Input: part model. Units: mm. Frame: model coordinates. A direction names the side the tool comes from. Give positions to 0.01 mm unless a question says otherwise; leave off trailing zeros. One line per item, written item: value.
Autodesk Fusion 360 part; units mm, degrees
sketch "Sketch1" plane through (0, 0, 0) normal (0, 1, 0) x (1, 0, 0)
  circle A0 centre (0, 0) radius 13
  circle A1 centre (0, 0) radius 3
  line L0 (0, 0) -> (0, 10)
  line L1 (0, 10) -> (3, 10)
  line L2 (3, 10) -> (3, 12)
  line L3 (3, 12) -> (-3, 12)
  line L4 (-3, 12) -> (-3, 10)
  line L5 (-3, 10) -> (3, 10)
  line L6 (-3, 10) -> (3, 10)
  line L7 (3, 10) -> (3, 6)
  line L8 (3, 6) -> (-3, 6)
  line L9 (-3, 6) -> (-3, 10)
  dimension "d1" = 26
  dimension "d2" = 6
extrude "Extrude1" add sketch "Sketch1" along normal blind 1 contours L0 L5 L6 L8 L9 | L0 L1 L5 L6 L7 L8
extrude "Extrude2" add sketch "Sketch1" along normal blind 6 contours L1 L2 L3 L4 L5 L6
extrude "Extrude3" add 1 faces at (-1, 6, -11.3333) along direction (0, 1, 0) blind 1
sketch "Sketch2" plane through (0, 0, -10) normal (0, 0, 1) x (1, 0, 0)
  line L0 (-3, 1) -> (3, 1)
  line L1 (3, 1) -> (3, 7)
  line L2 (3, 7) -> (-3, 7)
  line L3 (-3, 7) -> (-3, 1)
  line L4 (0, 7) -> (0, 5)
  circle A0 centre (0, 5) radius 0.5
  circle A1 centre (0, 5) radius 3
  circle A2 centre (0, 5) radius 1.5
  dimension "d9" = 2
  dimension "d10" = 1
  dimension "d23" = 3
extrude "Extrude4" cut sketch "Sketch2" against normal blind 5.8 contours A0
extrude "Extrude5" add 1 faces at (1, 1, -7.3333) along direction (0, 1, 0) blind 1
extrude "Extrude6" cut 1 faces at (1, 2, -7.3333) along direction (0, -1, 0) blind 0.5
extrude "Extrude7" cut sketch "Sketch2" against normal blind 1 contours A2 | L2 A1 picked at (-0.9591, 6.7853)
fillet "Fillet1" radius 2.3 1 edges at (0, 1.5, -10)
extrude "Extrude8" add 1 faces at (-0.0125, 6.4995, -11) along direction (0, 0, 1) blind 1
extrude "Extrude9" add 1 faces at (-1, 7, -10.6667) along direction (0, 1, 0) blind 1
extrude "Extrude10" cut sketch "Sketch2" against normal blind 1 contours A2
fillet "Fillet2" radius 3 2 edges at (-3, 8, -11) (3, 8, -11)
Item 1: Pin query (flat end, axial travel): P1, Ø1, axis at x = 0, z = -8.5, coming from the +Y side; P2, Ø1.8, axis at x = 0, y = 5, coming from the +Z side; P3, Ø3.5, axis at x = 0.5, y = 5.5, coming from the +Z side. Return the tip coordinate at first contact, or that it passes through.
Verdict:
P1: stops at y = 1.54
P2: stops at z = -11
P3: stops at z = -10
Item 2: Access query for faces 4 (the face through (0, 0, -9)), 5 (the face through (0, 1.5, -7)), 6 (the face through (-1.5, 5.07, -10.49)). Directions: +Z, -Z, +X, -X, +Y, -Y. A direction counts if a zero-diameter tool reaches every point of the face in a straight line with its end or side. Return the directions, or none.
Verdict:
face 4: +Z, -Z, +X, -X, -Y
face 5: +Z, +Y
face 6: +Z
Item 3: Material intervals for L1, parallel to Y at x = 0, z = -11.55; L2, parallel to X at y = 5, z = -10.7; L3, parallel to Y at x = 0.5, z = -8, sorted ascending.
Verdict:
L1: y = 0 to 4.5, 5.5 to 8
L2: x = -3 to -1.5, 1.5 to 3
L3: y = 0 to 1.5
Item 4: Draft query along X for faces 1 (the face through (0, 4, -12)), 2 (the face through (0, 4, -11)), 3 (the face through (-2.1, 7.14, -10.99)). Return one class per face: pulls with the +X half, pulls with the -X half, needs draft (parallel to the pull), parting line crosses it, or undercut.
Verdict:
face 1: needs draft
face 2: undercut
face 3: pulls with the -X half
